from build123d import *

# Parameters (mm, degrees)
SKETCH1_R           = 12.5
BOSS_EXTRUDE1_DEPTH = 27.0764
SKETCH2_R           = 11
BOSS_EXTRUDE2_DEPTH = 1.5
SKETCH3_R           = 12.5
BOSS_EXTRUDE3_DEPTH = 1.4
SKETCH4_R           = 6
BOSS_EXTRUDE4_DEPTH = 2.12
SKETCH5_R           = 2
BOSS_EXTRUDE5_DEPTH = 10
SKETCH6_W           = 2.63743778
SKETCH6_H           = 6.664381858
CUT_EXTRUDE1_DEPTH  = 8
SKETCH8_R           = 1.5
CUT_EXTRUDE2_DEPTH  = 6.35
SKETCH9_R           = 3.471368159
BOSS_EXTRUDE6_DEPTH = 5.5


with BuildPart() as part:
    # Sketch1 → Boss-Extrude1 (new body)
    with BuildSketch(Plane(origin=(0, 0, 0), x_dir=(0, 0, -1), z_dir=(1, 0, 0))):
        Circle(SKETCH1_R)
    extrude(amount=BOSS_EXTRUDE1_DEPTH)

    # Sketch2 → Boss-Extrude2 (add)
    with BuildSketch(Plane(origin=(27.0764, 0, 0), x_dir=(0, 0, -1), z_dir=(1, 0, 0))):
        Circle(SKETCH2_R)
    extrude(amount=BOSS_EXTRUDE2_DEPTH)

    # Sketch3 → Boss-Extrude3 (add)
    with BuildSketch(Plane(origin=(28.5764, 0, 0), x_dir=(0, 0, -1), z_dir=(1, 0, 0))):
        Circle(SKETCH3_R)
    extrude(amount=BOSS_EXTRUDE3_DEPTH)

    # Sketch4 → Boss-Extrude4 (add)
    with BuildSketch(Plane(origin=(29.9764, 0, 0), x_dir=(0, 0, -1), z_dir=(1, 0, 0))):
        Circle(SKETCH4_R)
    extrude(amount=BOSS_EXTRUDE4_DEPTH)

    # Sketch5 → Boss-Extrude5 (add)
    with BuildSketch(Plane(origin=(32.0964, 0, 0), x_dir=(0, 0, -1), z_dir=(1, 0, 0))):
        Circle(SKETCH5_R)
    extrude(amount=BOSS_EXTRUDE5_DEPTH)

    # Sketch6 → Cut-Extrude1 (cut)
    with BuildSketch(Plane(origin=(42.0964, 0, 0), x_dir=(0, 0, -1), z_dir=(1, 0, 0))):
        with Locations((2.91871889, -0.060449415)):
            Rectangle(SKETCH6_W, SKETCH6_H)
    extrude(amount=-CUT_EXTRUDE1_DEPTH, mode=Mode.SUBTRACT)

    # Sketch8 → Cut-Extrude2 (cut)
    with BuildSketch(Plane(origin=(29.9764, 0, 0), x_dir=(0, 0, -1), z_dir=(1, 0, 0))):
        with Locations((9, 0)):
            Circle(SKETCH8_R)
        with Locations((-9, 0)):
            Circle(SKETCH8_R)
    extrude(amount=-CUT_EXTRUDE2_DEPTH, mode=Mode.SUBTRACT)

    # Sketch9 → Boss-Extrude6 (add)
    with BuildSketch(Plane.ZY):
        with Locations((6.914557356, 0)):
            Circle(SKETCH9_R)
    extrude(amount=BOSS_EXTRUDE6_DEPTH)


solid = part.part
Input: part model. Units: mm. Frame: model coordinates. A direction names the side the tool comes from. Coordinates: 2 decimals unless noted, no trailing zeros. Loops run counter-clockwise (first coordinate to the right, second up) from the corner with the lowest first, then second, coordinate; pieces in that order, holes last.
Q1. Cut plane B-B (z = 0). Output: boundary loops of the cut face in (x, y), then the cut area to 3 significant figures.
Q2. Cut plane C-C (x = 9). Output: boundary loops of the cut face in (y, z).
Q3. Set-up query: faces 4 (the face through (26.8, -0.9, -7.8)), 5 (the face through (-5.5, 0, 7)), 6 (the face through (28.576, -10, -5)), 7 (the face through (38, 0, -1.6)), 8 (the face through (29.267, 3.755, -11.923)). Return all of +Z, -Z, +X, -X, +Y, -Y with unobstructed straight access to the full face (end or side cutting, diameter ignored); none if empty.
Q4. Draft query along X for faces 1 (the face through (42.096, 0, 0)), 2 (the face through (-2.71, -3.08, 8.52)), 3 (the face through (27.82, -10.74, 2.38)). Return one class per face: +X half, -X half, draft (parallel to the pull), parting line (faces both ways), or undercut.
Q5. Cut plane D-D (z = 4.5). Output: boundary loops of the cut face in (x, y).
Q6. Material intervals for line 1 (X direction, y = -6.25, z = -9.75); line 2 (X direction, y = 0, z = -6.75); line 3 (X direction, y = -3.25, z = 5), sorted ascending.
Q7. Contact query for flat-ended pins moving along their axis: pin 1 (4 mm diameter, centred on y = 10, z = 7, fed in from -X); pin 2 (2.5 mm diameter, centred on y = 0, z = 9, fed in from +X); pin 3 (2.5 mm diameter, centred on y = -0.5, z = -9.5, fed in from +X); pin 4 (7.5 mm diameter, centred on y = 1.5, z = 3, fed in from -X). Output: stop coordinate, or through.
Working result:
1. outline: (0, -12.5) - (27.08, -12.5) - (27.08, -11) - (28.58, -11) - (28.58, -12.5) - (29.98, -12.5) - (29.98, -6) - (32.1, -6) - (32.1, -2) - (42.1, -2) - (42.1, 2) - (32.1, 2) - (32.1, 6) - (29.98, 6) - (29.98, 12.5) - (28.58, 12.5) - (28.58, 11) - (27.08, 11) - (27.08, 12.5) - (0, 12.5) - close
1. area: 810 mm2
2. outline: circle Ø25 at (0, 0)
3. face 4: +X
3. face 5: +Z, -Z, -X, +Y, -Y
3. face 6: none
3. face 7: -Z, +X, +Y, -Y
3. face 8: +X, -X
4. face 1: +X half
4. face 2: draft
4. face 3: undercut
5. outline: (-5.5, -2.49) - (0, -2.49) - (0, -11.66) - (27.08, -11.66) - (27.08, -10.04) - (28.58, -10.04) - (28.58, -11.66) - (29.98, -11.66) - (29.98, -3.97) - (32.1, -3.97) - (32.1, 3.97) - (29.98, 3.97) - (29.98, 11.66) - (28.58, 11.66) - (28.58, 10.04) - (27.08, 10.04) - (27.08, 11.66) - (0, 11.66) - (0, 2.49) - (-5.5, 2.49) - close
6. line 1: x = 0 to 27.08, 28.58 to 29.98
6. line 2: x = 0 to 29.98
6. line 3: x = 0 to 32.1
7. pin 1: stops at x = 0
7. pin 2: stops at x = 23.63
7. pin 3: stops at x = 29.98
7. pin 4: stops at x = -5.5
